Source: CAD feature listing. Evaluate the final solid. Frame: model axes, mm. Face numbers are marked on the shaded views. A direction names the side the tool comes from. Give positions to 0.01 mm unless a question says otherwise; leave off trailing zeros. Loops run counter-clockwise (first coordinate to the right, second up) from the corner with the lowest first, then second, coordinate; pieces in that order, holes last. Notation, with made-up numbers: (52, 9.25) -> (80, 9.25) arc R10 cw to (80, 17.25) -> close; hole circle Ø11 at (-32, 8.25). An arc over 180 degrees is marked (long way). Put each result on its own line as item: value.
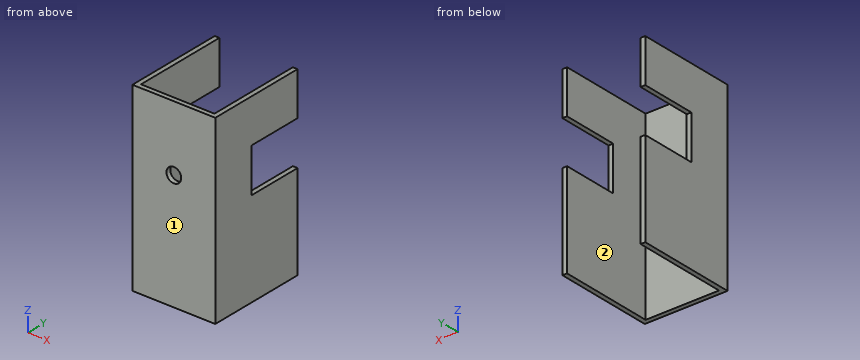
Autodesk Inventor part; units mm, degrees
ref_plane "YZ Plane" through (0, 0, 0) normal (1, 0, 0) x (0, 1, 0)
ref_plane "XZ Plane" through (0, 0, 0) normal (0, 1, 0) x (-1, 0, 0)
ref_plane "XY Plane" through (0, 0, 0) normal (0, 0, 1) x (1, 0, 0)
sketch "Sketch1" plane through (0, 0, 0) normal (0, 1, 0) x (-1, 0, 0)
  line L0 (-25, 62.04) -> (25, 62.04)
  line L1 (25, 62.04) -> (25, -62.04)
  line L2 (25, -62.04) -> (-25, -62.04)
  line L3 (-25, -62.04) -> (-25, 62.04)
  line L4 (-25, 62.04) -> (25, -62.04) construction
  line L5 (25, 62.04) -> (-25, -62.04) construction
  circle A0 centre (0, 17.59) radius 5
  point P0 (0, 0)
  dimension "d0" = 50
  dimension "d1" = 124.08
  dimension "d2" = 10
  dimension "d3" = 44.45
  dimension "d4" = 25
extrude "Extrusion1" add sketch "Sketch1" along normal blind 3.18
sketch "Sketch4" plane through (0, 0, 0) normal (0, 1, 0) x (-1, 0, 0)
  circle A0 centre (0, 17.59) radius 5
  line L0 (25, 62.04) -> (-25, 62.04)
  line L1 (-25, 62.04) -> (-25, -62.04)
  line L2 (-25, -62.04) -> (25, -62.04)
  line L3 (25, -62.04) -> (25, 62.04)
  line L4 (25, 62.04) -> (28.18, 62.04)
  line L5 (28.18, 62.04) -> (28.18, -62.04)
  line L6 (28.18, -62.04) -> (25, -62.04)
  line L7 (25, -62.04) -> (25, 62.04)
  line L8 (-25, 62.04) -> (-28.18, 62.04)
  line L9 (-28.18, 62.04) -> (-28.18, -62.04)
  line L10 (-28.18, -62.04) -> (-25, -62.04)
  line L11 (-25, -62.04) -> (-25, 62.04)
  point P0 (0, 0)
  dimension "d11" = 3.18
  dimension "d12" = 3.18
extrude "Extrusion3" add sketch "Sketch4" along normal blind 30 contours L4 L5 L6 L3 | L1 L10 L9 L8
sketch "Sketch5" plane through (0, 30, 0) normal (0, 1, 0) x (1, 0, 0)
  line L0 (-25, -62.04) -> (-25, 62.04)
  line L1 (-25, 62.04) -> (-28.18, 62.04)
  line L2 (-28.18, 62.04) -> (-28.18, -62.04)
  line L3 (-28.18, -62.04) -> (-25, -62.04)
  line L4 (25, -62.04) -> (28.18, -62.04)
  line L5 (28.18, -62.04) -> (28.18, 62.04)
  line L6 (28.18, 62.04) -> (25, 62.04)
  line L7 (25, 62.04) -> (25, -62.04)
  line L8 (-25, 62.04) -> (-25, -62.04)
  line L9 (-28.18, -62.04) -> (-25, -62.04)
  line L10 (-25, -62.04) -> (-25, -32.5)
  line L11 (-25, -32.5) -> (-28.18, -32.5)
  line L12 (-28.18, -32.5) -> (-28.18, -62.04)
  line L13 (-28.18, 62.04) -> (28.18, 62.04)
  line L14 (-28.18, 62.04) -> (-25, 62.04)
  line L15 (-25, 62.04) -> (-25, -2.5)
  line L16 (-25, -2.5) -> (-28.18, -2.5)
  line L17 (-28.18, -2.5) -> (-28.18, 62.04)
  line L18 (28.18, -62.04) -> (28.18, 62.04)
  line L19 (25, -62.04) -> (28.18, -62.04)
  line L20 (28.18, -62.04) -> (28.18, -32.5)
  line L21 (28.18, -32.5) -> (25, -32.5)
  line L22 (25, -32.5) -> (25, -62.04)
  line L23 (25, -62.04) -> (25, 62.04)
  line L24 (28.18, 62.04) -> (25, 62.04)
  line L25 (25, 62.04) -> (25, -2.5)
  line L26 (25, -2.5) -> (28.18, -2.5)
  line L27 (28.18, -2.5) -> (28.18, 62.04)
  point P0 (0, 0)
  dimension "d15" = 29.54
  dimension "d16" = 64.54
  dimension "d17" = 29.54
  dimension "d18" = 64.54
extrude "Extrusion4" add sketch "Sketch5" along normal blind 38.18 contours L3 L2 L11 L0 | L16 L2 L1 L0
sketch "Sketch6" plane through (0, 30, 0) normal (0, 1, 0) x (1, 0, 0)
  line L0 (25, -62.04) -> (28.18, -62.04)
  line L1 (28.18, -62.04) -> (28.18, 62.04)
  line L2 (28.18, 62.04) -> (25, 62.04)
  line L3 (25, 62.04) -> (25, -62.04)
  line L4 (28.18, -62.04) -> (28.18, 62.04)
  line L5 (25, -62.04) -> (25, 62.04)
  line L6 (28.18, -62.04) -> (25, -62.04)
  line L7 (25, -62.04) -> (25, -32.5)
  line L8 (25, -32.5) -> (28.18, -32.5)
  line L9 (28.18, -32.5) -> (28.18, -62.04)
  line L10 (28.18, 62.04) -> (25, 62.04)
  line L11 (25, 62.04) -> (25, -2.5)
  line L12 (25, -2.5) -> (28.18, -2.5)
  line L13 (28.18, -2.5) -> (28.18, 62.04)
  point P0 (0, 0)
  dimension "d21" = 29.54
  dimension "d22" = 64.54
extrude "Extrusion5" add sketch "Sketch6" along normal blind 38.18 contours L3 L8 L1 L0 | L3 L2 L1 L12
properties part number "Hombro_base"
(1) First-contact query: P1, Ø25, axis at x = -5, z = 3.5, coming from the +Y side; P2, Ø1.6, axis at x = -27.5, z = 11.5, coming from the +Y side. Flat tips, straight axial feed; report the tip coordinate or a pass-through.
Calculated:
P1: stops at y = 3.18
P2: stops at y = 30
(2) Section C-C on z = -47.5. Return loops of the section in (x, y).
Calculated:
outline: (-28.18, 0) -> (28.18, 0) -> (28.18, 68.18) -> (25, 68.18) -> (25, 3.18) -> (-25, 3.18) -> (-25, 68.18) -> (-28.18, 68.18) -> close
(3) Section D-D on x = 21.5. Return loops of the section in (y, z), then the cut area to 3 significant figures.
Calculated:
outline: (0, -62.04) -> (3.18, -62.04) -> (3.18, 62.04) -> (0, 62.04) -> close
area: 395 mm²
(4) Reachability of the marked faces 1 and 2 from +Z, -Z, +X, -X, +Y, -Y: full face, straight path, thin tool, end or side. Return the list, or none.
Calculated:
face 1: +Z, -Z, +X, -X, -Y
face 2: +Z, -Z, +Y
(5) Section A-A on z = 17.59. Return loops of the section in (x, y), then the cut area to 3 significant figures.
Calculated:
outline: (-28.18, 0) -> (-5, 0) -> (-5, 3.18) -> (-25, 3.18) -> (-25, 30) -> (-28.18, 30) -> close; (5, 0) -> (28.18, 0) -> (28.18, 30) -> (25, 30) -> (25, 3.18) -> (5, 3.18) -> close
area: 318 mm²
(6) Line query: probe 1 along X at (y, z) = (46, 43); probe 2 along Z at (x, y) = (0, 2.35); probe 3 along Y at (x, z) = (-1.5, 30). Output: solid intervals per line, ascending. Write a range as from..to.
Calculated:
probe 1: x = -28.18..-25, 25..28.18
probe 2: z = -62.04..12.59, 22.59..62.04
probe 3: y = 0..3.18
(7) Section B-B on x = 0. Return loops of the section in (y, z), then the cut area to 3 significant figures.
Calculated:
outline: (0, -62.04) -> (3.18, -62.04) -> (3.18, 12.59) -> (0, 12.59) -> close; (0, 22.59) -> (3.18, 22.59) -> (3.18, 62.04) -> (0, 62.04) -> close
area: 363 mm²
